Work out the finished part from the listing and answer in its coordinate system (mm). A direction names the side the tool comes from. Give positions to 0.01 mm unless a question says otherwise; leave off trailing zeros. Loops run counter-clockwise (first coordinate to the right, second up) from the corner with the lowest first, then second, coordinate; pieces in that order, holes last. Notation, with made-up numbers: (3, -4) - (45, -4) arc R30 ccw to (45, 26) - close; hole circle Ø10 at (-31.5, -29). An arc over 180 degrees is marked (long way). Use one line per item in the form item = value. Start each with the question number.
from build123d import *

# Parameters (mm, degrees)
BOSS_EXTRUDE1_DEPTH = 5
SKETCH2_W           = 6
SKETCH2_H           = 5
BOSS_EXTRUDE2_DEPTH = 1


with BuildPart() as part:
    # Sketch1 → Boss-Extrude1 (new body)
    with BuildSketch(Plane(origin=(0, 0, 0), x_dir=(1, 0, 0), z_dir=(0, 1, 0))):
        Polygon((-22, -1), (22, -1), (22, -4.5), (25, -4.5), (25, -0.5), (25, 0.5), (-25, 0.5), (-25, -0.5), (-25, -4.5), (-22, -4.5), align=None)
    extrude(amount=BOSS_EXTRUDE1_DEPTH)

    # Sketch2 → Boss-Extrude2 (add)
    with BuildSketch(Plane.XY.offset(4.5)):
        with Locations((-25, 2.5)):
            Rectangle(SKETCH2_W, SKETCH2_H)
    boss_extrude2 = extrude(amount=-BOSS_EXTRUDE2_DEPTH)

    # Mirror1: Boss-Extrude2 across plane
    add(boss_extrude2.mirror(Plane(origin=(0, 0, 0), x_dir=(0, 0, 1), z_dir=(1, 0, 0))))


solid = part.part
1) A cutting plane is placed at B-B (y = 0.55). Give the vertices of the cut face in (x, z).
2) A cutting plane is placed at C-C (x = 18.5). Give the vertices of the cut face in (y, z), plus the area to 3 significant figures.
3) Find the intervals of material crossed by probe 1 along X at (y, z) = (1.1, 1.7); probe 2 along X at (y, z) = (2.05, 4.2); probe 3 along Z at (x, y) = (4.5, 2.55), in increasing order.
4) A cutting plane is placed at A-A (z = 1.6). Give the vertices of the cut face in (x, y).
5) A tool of negligible diameter and unlimited length cuts with its end or side. For faces 1 (the flat face through (-27, 3, 3.5)), 2 (the flat face through (-6, 5, 0)), 3 (the flat face through (22, 2, 3)), 4 (the flat face through (25, 2, 2)), from which of +Z, -Z, +X, -X, +Y, -Y can it reach the whole face along a straight path? Write none if from no direction.
6) Flat-ended cylindrical pins translate along their axes: pin 1 Ø0.9 at (x, y) = (-26.5, 3) entering from -Z; pin 2 Ø1.8 at (y, z) = (1.5, 2) entering from +X; pin 3 Ø2 at (y, z) = (3, 1.5) entering from -X. Find the tip coordinate at first contact, or state that the pin passes through.
Answer sheet:
q1.outline = (-28, 3.5) - (-25, 3.5) - (-25, -0.5) - (25, -0.5) - (25, 3.5) - (28, 3.5) - (28, 4.5) - (22, 4.5) - (22, 1) - (-22, 1) - (-22, 4.5) - (-28, 4.5) - close
q2.outline = (0, -0.5) - (5, -0.5) - (5, 1) - (0, 1) - close
q2.area = 7.50 mm²
q3.probe_1 = -25 to -22, 22 to 25
q3.probe_2 = -28 to -22, 22 to 28
q3.probe_3 = -0.5 to 1
q4.outline = (-25, 0) - (-22, 0) - (-22, 5) - (-25, 5) - close; (22, 0) - (25, 0) - (25, 5) - (22, 5) - close
q5.face_1 = -Z, -X, +Y, -Y
q5.face_2 = +Z, -Z, +X, -X, +Y
q5.face_3 = +Z, +Y, -Y
q5.face_4 = -Z, +X, +Y, -Y
q6.pin_1 = 3.5
q6.pin_2 = 25
q6.pin_3 = -25
